Read the model definition and answer for the solid it produces. Units are mm, in the model's axes. A direction names the side the tool comes from. Coordinates: 2 decimals unless noted, no trailing zeros. Loops run counter-clockwise (first coordinate to the right, second up) from the corner with the lowest first, then second, coordinate; pieces in that order, holes last. Notation, with made-up numbers: (-13.5, -8) -> (4.5, -8) arc R13 ccw to (4.5, 4) -> close; hole circle Ø4 at (-12.75, 41.5). An arc over 180 degrees is marked (long way). Answer as CSV lines item,"result".
```python
from build123d import *

# Parameters (mm, degrees)
SKETCH1_W                 = 63.5
SKETCH1_H                 = 82.55
BOSS_EXTRUDE1_DEPTH       = 57.15
SHELL1_T                  = 3.175
SKETCH3_R                 = 3.175
BOSS_EXTRUDE2_DEPTH       = 3.175
SKETCH2_R                 = 0.9525
CUT_EXTRUDE1_DEPTH        = 6.35
CUT_EXTRUDE1_DEPTH_BACK   = 0.0127
FILLET1_R                 = 2.54
SKETCH4_W                 = 12.192
SKETCH4_H                 = 10.922
CUT_EXTRUDE2_DEPTH        = 123.721040372
SKETCH5_W                 = 14.605
SKETCH5_H                 = 19.685
CUT_EXTRUDE3_DEPTH        = 125.474578228
F_4_40_TAPPED_HOLE1_D     = 2.2606
F_4_40_TAPPED_HOLE1_DEPTH = 6.35
F_4_40_TAPPED_HOLE1_TIP   = 0.679152758


with BuildPart() as part:
    # Sketch1 → Boss-Extrude1 (new body)
    with BuildSketch(Plane(origin=(0, 0, 0), x_dir=(1, 0, 0), z_dir=(0, 1, 0))):
        with Locations((31.75, -41.275)):
            Rectangle(SKETCH1_W, SKETCH1_H)
    extrude(amount=BOSS_EXTRUDE1_DEPTH)

    # Shell1
    shell1_openings = [part.faces().sort_by_distance(p)[0] for p in [
        (31.75, 57.15, 41.275),
    ]]
    offset(amount=SHELL1_T, openings=shell1_openings, kind=Kind.INTERSECTION)

    # Sketch3 → Boss-Extrude2 (add)
    with BuildSketch(Plane(origin=(0, 0, 0), x_dir=(1, 0, 0), z_dir=(0, 1, 0))):
        with Locations(Location((12.827, -68.58, 0), (0, 0, 270))):
            Circle(SKETCH3_R)
        with Locations(Location((40.132, -68.58, 0), (0, 0, 270))):
            Circle(SKETCH3_R)
        with Locations(Location((56.007, -17.78, 0), (0, 0, 270))):
            Circle(SKETCH3_R)
    extrude(amount=BOSS_EXTRUDE2_DEPTH)

    # Sketch2 → Cut-Extrude1 (cut, two sides)
    with BuildSketch(Plane(origin=(0, 0, 0), x_dir=(1, 0, 0), z_dir=(0, 1, 0))) as cut_extrude1_sk:
        with Locations(Location((12.827, -68.58, 0), (0, 0, 270))):
            Circle(SKETCH2_R)
        with Locations(Location((40.132, -68.58, 0), (0, 0, 270))):
            Circle(SKETCH2_R)
        with Locations(Location((56.007, -17.78, 0), (0, 0, 270))):
            Circle(SKETCH2_R)
    extrude(amount=CUT_EXTRUDE1_DEPTH, mode=Mode.SUBTRACT)
    extrude(cut_extrude1_sk.sketch, amount=-CUT_EXTRUDE1_DEPTH_BACK, mode=Mode.SUBTRACT)

    # Fillet1
    fillet1_edges = [part.edges().sort_by_distance(p)[0] for p in [
        (0, 28.575, 0),
        (0, 28.575, 82.55),
        (63.5, 28.575, 82.55),
        (63.5, 28.575, 0),
        (-3.175, 26.9875, -3.175),
        (66.675, 26.9875, -3.175),
        (66.675, 26.9875, 85.725),
        (-3.175, 26.9875, 85.725),
    ]]
    fillet(fillet1_edges, radius=FILLET1_R)

    # Sketch4 → Cut-Extrude2 (cut, through all)
    with BuildSketch(Plane.XY):
        with Locations((42.799, 10.287)):
            Rectangle(SKETCH4_W, SKETCH4_H)
    extrude(amount=-CUT_EXTRUDE2_DEPTH, mode=Mode.SUBTRACT)

    # Sketch5 → Cut-Extrude3 (cut, through all)
    with BuildSketch(Plane(origin=(66.675, 0, 0), x_dir=(0, 0, -1), z_dir=(1, 0, 0))):
        with Locations((-37.7825, 31.0515)):
            Rectangle(SKETCH5_W, SKETCH5_H)
    extrude(amount=-CUT_EXTRUDE3_DEPTH, mode=Mode.SUBTRACT)

    # #4-40 Tapped Hole1
    with Locations(Plane(origin=(0, 57.15, 0), x_dir=(1, 0, 0), z_dir=(0, 1, 0))):
        with Locations((64.135, -83.185), (-0.635, -83.185), (-0.635, 0.635), (64.135, 0.635)):
            Hole(F_4_40_TAPPED_HOLE1_D / 2, depth=F_4_40_TAPPED_HOLE1_DEPTH)
            with Locations((0, 0, -(F_4_40_TAPPED_HOLE1_DEPTH + F_4_40_TAPPED_HOLE1_TIP / 2))):  # 118° drill point
                Cone(0, F_4_40_TAPPED_HOLE1_D / 2, F_4_40_TAPPED_HOLE1_TIP, mode=Mode.SUBTRACT)


solid = part.part
```
Q1. A cutting plane is placed at B-B, the plane z = 33. Write down the section's boundary in (x, y) (3 decimals), and give its area (3 significant figures).
Results:
outline,"(-3.175, -3.175) -> (66.675, -3.175) -> (66.675, 21.209) -> (63.5, 21.209) -> (63.5, 0) -> (0, 0) -> (0, 21.209) -> (-3.175, 21.209) -> close; (-3.175, 40.894) -> (0, 40.894) -> (0, 57.15) -> (-3.175, 57.15) -> close; (63.5, 40.894) -> (66.675, 40.894) -> (66.675, 57.15) -> (63.5, 57.15) -> close"
area,"460 mm²"
Q2. For faces 1 (the face through (66.675, 20, 42)), 2 (the face through (65.264, 53.931, -0.685)), 3 (the face through (-2, 21.209, 38)), 4 (the face through (43, 4.826, -2)), determine the directions among +Z, -Z, +X, -X, +Y, -Y from which every point of the face is accessible in a straight line to the end or side of a thin tool.
Results:
face 1,"+Z, -Z, +X, +Y, -Y"
face 2,"+Y"
face 3,"+X, -X"
face 4,"-Z"
Q3. A cutting plane is placed at A-A, the plane x = 45. Write down the section's boundary in (y, z) (3 decimals).
Results:
outline,"(-3.175, -3.175) -> (4.826, -3.175) -> (4.826, 0) -> (0, 0) -> (0, 82.55) -> (57.15, 82.55) -> (57.15, 85.725) -> (-3.175, 85.725) -> close; (15.748, -3.175) -> (57.15, -3.175) -> (57.15, 0) -> (15.748, 0) -> close"
Q4. Given pin 1 Ø2 at (x, z) = (40.5, 68.5) entering from +Y (3 decimals); pin 2 Ø1.5 at (x, z) = (12.827, 68.58) entering from +Y; pin 3 Ø1.6 at (y, z) = (10.5, -2) entering from +X; pin 4 Ø2.5 at (x, y) = (-1, 32) entering from -Z (3 decimals), each flat-ended and moving along its own axis, determine where each tip first touches the part or whether it passes through.
Results:
pin 1,"stops at y = 3.175"
pin 2,"stops at y = -0.01"
pin 3,"stops at x = 66.61"
pin 4,"stops at z = -3.175"
Q5. A cutting plane is placed at C-C, the plane x = 26. Write down the section's boundary in (y, z) (3 decimals), and give its area (3 significant figures).
Results:
outline,"(-3.175, -3.175) -> (57.15, -3.175) -> (57.15, 0) -> (0, 0) -> (0, 82.55) -> (57.15, 82.55) -> (57.15, 85.725) -> (-3.175, 85.725) -> close"
area,"645 mm²"
Q6. A cutting plane is placed at D-D, the plane z = 55. Write down the section's boundary in (x, y) (3 decimals).
Results:
outline,"(-3.175, -3.175) -> (66.675, -3.175) -> (66.675, 57.15) -> (63.5, 57.15) -> (63.5, 0) -> (0, 0) -> (0, 57.15) -> (-3.175, 57.15) -> close"
Q7. Find the intervals of material crossed by probe 1 along Z at (x, y) = (53.5, 40.5) (3 decimals); probe 2 along X at (y, z) = (44.5, 27) (3 decimals); probe 3 along Y at (x, z) = (39.5, 23) (3 decimals), in increasing order. Write a range as [from, to].
Results:
probe 1,"z = [-3.175, 0], [82.55, 85.725]"
probe 2,"x = [-3.175, 0], [63.5, 66.675]"
probe 3,"y = [-3.175, 0]"
Q8. For a pull along X with two mould halves and no side action, classify faces 5 (the face through (-2.41, 26.57, -2.45)), 6 (the face through (-2, 31, 30.48)), 7 (the face through (31, 28, 0)) as pulls with the +X half, pulls with the -X half, needs draft (parallel to the pull), parting line crosses it, or undercut.
Results:
face 5,"pulls with the -X half"
face 6,"needs draft"
face 7,"undercut"
